The drawing under review shows one solid part. Ordinate dimensions are in mm from its lowest x, y, z. Round coordinates to 2 decimals unless told otherwise and drop trailing zeros. Write each loop counter-clockwise with the first axis right and the second up, starting at its lowest first coordinate (ties: lowest second). Pieces come first, ordered by that corner, then holes. Notation, with made-up numbers: (-37, -17) -> (5, -17) arc R9 cw to (5, -4) -> close; hole circle Ø1 at (-30, 11). An arc over 180 degrees is marked (long way). Answer in a Markdown table with one row per item. Add a question column.
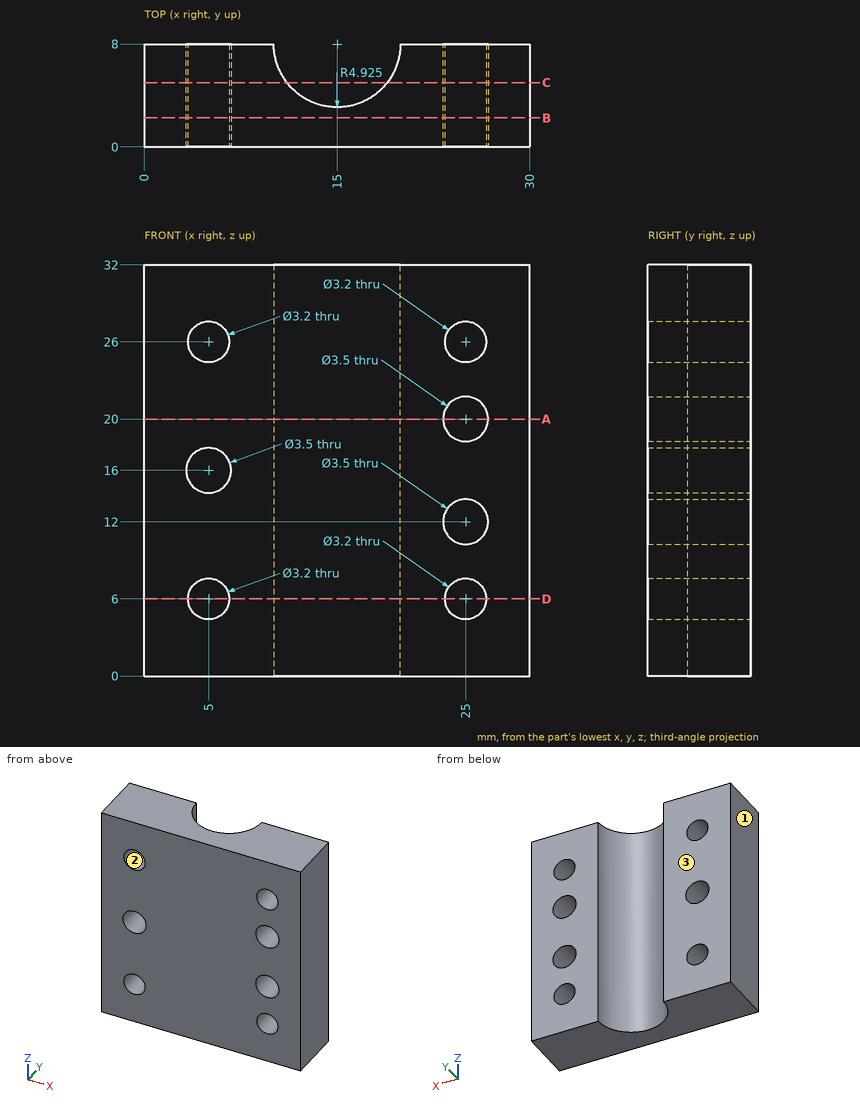
1. For L1, parallel to X at y = 2, z = 6; L2, parallel to Z at x = 25, y = 2.25; L3, parallel to X at y = 6, z = 6, list the stretches that pass through material, from the lowest coordinate up.
2. Mouldability with a two-part tool opening along X and no side actions: class the marked faces 1, 2 and 3 as pulls with the +X half, pulls with the -X half, needs draft (parallel to the pull), parting line crosses it, or undercut.
3. Add section C-C on y = 5. State how many separate pieces and enclosed holes the cut face has, plus the area to 3 significant figures.
4. Insertion check: pin 1 Ø2.5 at (x, z) = (25, 26) entering from +Y. The pin has a flat end and moves straight along its axis. Give the tip position at first contact, or say it passes through.
5. Add section B-B on y = 2.25. Write out the cut boundary in (x, z).
6. Add section A-A on z = 20. Write out the cut boundary in (x, y) (3 decimals).
7. Add section D-D on z = 6. Write out the cut boundary in (x, y) (3 decimals), plus the area to 3 significant figures.
Filled in:
| question | item | result |
|---|---|---|
| 1 | L1 | 0 to 3.4, 6.6 to 23.4, 26.6 to 30 |
| 1 | L2 | 0 to 4.4, 7.6 to 10.25, 13.75 to 18.25, 21.75 to 24.4, 27.6 to 32 |
| 1 | L3 | 0 to 3.4, 6.6 to 10.5, 19.5 to 23.4, 26.6 to 30 |
| 2 | face 1 | pulls with the -X half |
| 2 | face 2 | undercut |
| 2 | face 3 | needs draft |
| 3 | separate pieces | 2 |
| 3 | enclosed holes | 7 |
| 3 | area | 649 mm² |
| 4 | pin 1 | through |
| 5 | outline | (0, 0) -> (30, 0) -> (30, 32) -> (0, 32) -> close; hole circle Ø3.5 at (5, 16); hole circle Ø3.2 at (5, 6); hole circle Ø3.2 at (5, 26); hole circle Ø3.5 at (25, 12); hole circle Ø3.5 at (25, 20); hole circle Ø3.2 at (25, 6); hole circle Ø3.2 at (25, 26) |
| 6 | outline | (0, 0) -> (23.25, 0) -> (23.25, 8) -> (19.925, 8) arc R4.925 cw to (10.075, 8) -> (0, 8) -> close; (26.75, 0) -> (30, 0) -> (30, 8) -> (26.75, 8) -> close |
| 7 | outline | (0, 0) -> (3.4, 0) -> (3.4, 8) -> (0, 8) -> close; (6.6, 0) -> (23.4, 0) -> (23.4, 8) -> (19.925, 8) arc R4.925 cw to (10.075, 8) -> (6.6, 8) -> close; (26.6, 0) -> (30, 0) -> (30, 8) -> (26.6, 8) -> close |
| 7 | area | 151 mm² |
